Geometry check sheet. Reference: the model listing, model coordinates, mm. Round coordinates to 2 decimals unless told otherwise and drop trailing zeros. Write each loop counter-clockwise with the first axis right and the second up, starting at its lowest first coordinate (ties: lowest second). Pieces come first, ordered by that corner, then holes. Notation, with made-up numbers: (46, 39.25) - (85, 39.25) arc R24 cw to (85, 73.25) - close; hole circle Ø9 at (33, 53.5). An arc over 180 degrees is marked (long way). Return JSON: item names as keys, results as strings. Group by question number.
Autodesk Inventor part; units mm, degrees
ref_plane "YZ Plane" through (0, 0, 0) normal (1, 0, 0) x (0, 1, 0)
ref_plane "XZ Plane" through (0, 0, 0) normal (0, 1, 0) x (-1, 0, 0)
ref_plane "XY Plane" through (0, 0, 0) normal (0, 0, 1) x (1, 0, 0)
sketch "Sketch1" plane through (0, 0, 0) normal (1, 0, 0) x (0, 1, 0)
  line L0 (-12.7, 25.4) -> (-12.7, -25.4)
  line L1 (-12.7, -25.4) -> (12.7, -25.4)
  line L2 (12.7, -25.4) -> (12.7, 25.4)
  line L3 (12.7, 25.4) -> (-12.7, 25.4)
  line L4 (-12.7, 25.4) -> (12.7, -25.4) construction
  line L5 (-12.7, -25.4) -> (12.7, 25.4) construction
  line L6 (-9.525, 22.225) -> (-9.525, -22.225)
  line L7 (-9.525, -22.225) -> (9.525, -22.225)
  line L8 (9.525, -22.225) -> (9.525, 22.225)
  line L9 (9.525, 22.225) -> (-9.525, 22.225)
  line L10 (-9.525, 22.225) -> (9.525, -22.225) construction
  line L11 (-9.525, -22.225) -> (9.525, 22.225) construction
  point P0 (0, 0)
  dimension "d0" = 25.4
  dimension "d1" = 50.8
  dimension "d2" = 3.175
  dimension "d3" = 3.175
extrude "Extrusion1" add sketch "Sketch1" along normal mid plane 542.925
equation "\"d0\" = width"
equation "\"d1\" = height"
equation "\"d2\" = wallThickness"
equation "\"d3\" = wallThickness"
equation "\"d4\" = length"
equation "\"width\" = 25.4"
equation "\"height\" = 50.8"
equation "\"length\" = 542.925"
equation "\"wallThickness\" = 3.175"
properties part number "1x2_alumTubing" material "Aluminum 6061"
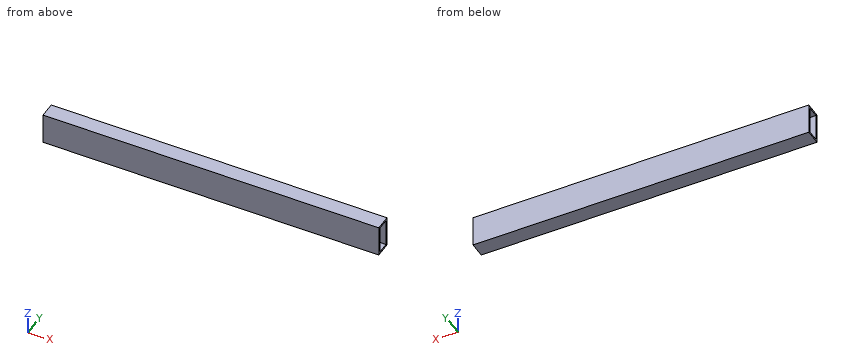
1. Section check C-C (x = 186). Enter the section's corners in (y, z) (3 decimals).
2. Section check B-B (z = 14). Enter the section's corners in (x, y) (1 decimal).
3. Material ranges on line 1 along Z through (x, y) = (16, 9.25) (3 decimals); line 2 along Y through (x, z) = (82, -4.5) (3 decimals), recorded low to high.
4. Section check A-A (y = -2). Enter the section's corners in (x, z) (1 decimal), and give its area (3 significant figures).
Result sheet:
{
 "1": {"outline": "(-12.7, -25.4) - (12.7, -25.4) - (12.7, 25.4) - (-12.7, 25.4) - close; hole (-9.525, -22.225) - (9.525, -22.225) - (9.525, 22.225) - (-9.525, 22.225) - close"},
 "2": {"outline": "(-271.5, -12.7) - (271.5, -12.7) - (271.5, -9.5) - (-271.5, -9.5) - close; (-271.5, 9.5) - (271.5, 9.5) - (271.5, 12.7) - (-271.5, 12.7) - close"},
 "3": {"line 1": "z = -25.4 to -22.225, 22.225 to 25.4", "line 2": "y = -12.7 to -9.525, 9.525 to 12.7"},
 "4": {"outline": "(-271.5, -25.4) - (271.5, -25.4) - (271.5, -22.2) - (-271.5, -22.2) - close; (-271.5, 22.2) - (271.5, 22.2) - (271.5, 25.4) - (-271.5, 25.4) - close", "area": "3,450 mm²"}
}
